The model under review builds one solid part; all positions refer to its coordinate system, in mm. A direction names the side the tool comes from. Round coordinates to 2 decimals unless told otherwise and drop trailing zeros. Order: outer loops, then holes, each group sorted by start corner. A loop starts at its lowest first (then second) coordinate and runs counter-clockwise, first axis right, second up.
```python
from build123d import *

# Parameters (mm, degrees)
F0_R     = 76.2
F2_R     = 50.8
F4_DEPTH = 12.7
F5_R     = 6.35
F8_W     = 1.5875
F8_H     = 152.4


with BuildPart() as f3:
    # F0 (on Top) → F3 section 0
    with BuildSketch(Plane.XY):
        Circle(F0_R)
    # F2 (on offset) → F3 section 1
    with BuildSketch(Plane.XY.offset(25.4)):
        Circle(F2_R)
    loft()

    # F0 (on Top) → F4 (join)
    with BuildSketch(Plane.XY):
        Circle(F0_R)
    extrude(amount=-F4_DEPTH)

    # F7: sweep along a path in F6
    with BuildLine(Plane.XZ) as f7_path:
        Line((0, 25.4), (0, 12.7))
        ThreePointArc((0, 12.7), (-3.7197438789, 3.7197438789), (-12.7, 0))
        Line((-12.7, 0), (-82.2157882963, 0))
    # F5 (on face) → F7 (sweep, cut)
    with BuildSketch(Plane.XY.offset(25.4)):
        Circle(F5_R)
    sweep(path=f7_path.line, mode=Mode.SUBTRACT)

    # F8 (on Front) → F9 (revolve)
    with BuildSketch(Plane.XZ):
        with Locations((7.14375, 101.6)):
            Rectangle(F8_W, F8_H)
    revolve(axis=Axis((0, 0, 88.9), (0, 0, 1)))


solid = f3.part
```
(1) Consider section A-A (z = 17.5). Write out the cut boundary in (x, y), and give its area (3 significant figures).
Data:
outline: circle Ø117.4 at (0, 0); hole circle Ø12.7 at (0, 0)
area: 10,700 mm2
(2) Insertion check: pin 1 (12 mm diameter, centred on x = 38, y = -11, fed in from +Z). The pin has a flat end and moves straight along its axis. Give the tip position at first contact, or say it passes through.
Data:
pin 1: stops at z = 25.4
(3) To check wall thickness, follow probe 1 along Y at (x, z) = (0, 100); probe 2 along Z at (x, y) = (34, 19.5); probe 3 along Z at (x, y) = (-62, 0). State the ranges of each line that lie inside material, in increasing order.
Data:
probe 1: y = -7.94 to -6.35, 6.35 to 7.94
probe 2: z = -12.7 to 25.4
probe 3: z = -12.7 to -6.35, 6.35 to 14.2
(4) Draft analysis for pull direction Y (two halves, no side actions). For faces 1 (the cylindrical face through (-44.894, -1.907, -6.057)), 2 (the conical face through (48.066, -19.929, 24.167)), 3 (the flat face through (11, 1, 25.4)), state which applies: pulls with the +Y half, pulls with the -Y half, needs draft (parallel to the pull), parting line crosses it, or undercut.
Data:
face 1: undercut
face 2: parting line crosses it
face 3: needs draft
(5) For faces 4 (the cylindrical face through (72.68, 22.89, -6.26)), 5 (the cylindrical face through (-1.38, -6.2, 96.41)), list the 3-axis set-ups (+Z, -Z, +X, -X, +Y, -Y) from which the entire face can be reached by the end or side of a thin tool; tool diameter is ignored.
Data:
face 4: +Z, -Z
face 5: +Z
